```python
from build123d import *

# Parameters (mm, degrees)
SKETCH1_R           = 64
BOSS_EXTRUDE1_DEPTH = 7
SKETCH2_R           = 37.5
SKETCH2_R_2         = 32.5
BOSS_EXTRUDE2_DEPTH = 12
SKETCH3_R           = 12.5
CUT_EXTRUDE1_DEPTH  = 92.301697684
FILLET1_R           = 2
SKETCH17_R          = 13.5
BOSS_EXTRUDE3_DEPTH = 30


with BuildPart() as part:
    # Sketch1 → Boss-Extrude1 (new body)
    with BuildSketch(Plane(origin=(0, 0, 0), x_dir=(1, 0, 0), z_dir=(0, 1, 0))):
        with Locations(Location((0, 0, 0), (0, 0, 270))):
            Circle(SKETCH1_R)
    extrude(amount=BOSS_EXTRUDE1_DEPTH)

    # Sketch2 → Boss-Extrude2 (add)
    with BuildSketch(Plane(origin=(0, 7, 0), x_dir=(1, 0, 0), z_dir=(0, 1, 0))):
        with Locations(Location((0, 0, 0), (0, 0, 270))):
            Circle(SKETCH2_R)
        with Locations(Location((0, 0, 0), (0, 0, 270))):
            Circle(SKETCH2_R_2, mode=Mode.SUBTRACT)
    extrude(amount=BOSS_EXTRUDE2_DEPTH)

    # Sketch3 → Cut-Extrude1 (cut, through all)
    with BuildSketch(Plane(origin=(0, 7, 0), x_dir=(1, 0, 0), z_dir=(0, 1, 0))):
        with Locations(Location((0, 0, 0), (0, 0, 270))):
            Circle(SKETCH3_R)
    extrude(amount=-CUT_EXTRUDE1_DEPTH, mode=Mode.SUBTRACT)

    # Fillet1
    fillet1_edges = [part.edges().sort_by_distance(p)[0] for p in [
        (0, 0, -64),
        (0, 7, -64),
        (0, 19, -37.5),
        (0, 19, -32.5),
    ]]
    fillet(fillet1_edges, radius=FILLET1_R)

    # Sketch17 → Boss-Extrude3 (add)
    with BuildSketch(Plane(origin=(0, 7, 0), x_dir=(1, 0, 0), z_dir=(0, 1, 0))):
        with Locations(Location((0, 35, 0), (0, 0, 359.939369671))):
            Circle(SKETCH17_R)
    extrude(amount=BOSS_EXTRUDE3_DEPTH)


solid = part.part
```
Geometry: final body of the model. Coordinates: model frame, mm. A direction names the side the tool comes from. Round coordinates to 2 decimals unless told otherwise and drop trailing zeros. Write each loop counter-clockwise with the first axis right and the second up, starting at its lowest first coordinate (ties: lowest second). Pieces come first, ordered by that corner, then holes.
Item 1: Material intervals for L1, parallel to X at y = 11.75, z = 0; L2, parallel to X at y = 4.5, z = 0; L3, parallel to Y at x = 1, z = -53.5, sorted ascending.
Item 2: Set-up query: faces 4 (the face through (-27, 7, 27)), 5 (the face through (3.755, 3.549, 11.923)). Return all of +Z, -Z, +X, -X, +Y, -Y with unobstructed straight access to the full face (end or side cutting, diameter ignored); none if empty.
Item 3: Section query A-A (z = 0). Return loops of the section in (x, y).
Item 4: Section query C-C (y = 15). Return loops of the section in (x, z).
Item 5: Pin query (flat end, axial travel): P1, Ø10, axis at y = 10.5, z = 5, coming from the -X side; P2, Ø3, axis at x = -31, z = -50, coming from the +Y side; P3, Ø8, axis at x = -4, y = 14.5, coming from the -Z side. Return the tip coordinate at first contact, or that it passes through.
Item 6: Section query D-D (y = 28.5). Return loops of the section in (x, z).
Item 7: Section query B-B (x = 0). Return loops of the section in (y, z).
Item 8: Mould query, pull axis Z, two halves, no side actions, for faces 1 (the face through (-13, 0, -1)), 2 (the face through (-1.249, 11.93, 32.476)), 3 (the face through (-62.48, 3.48, -13.87)). Classes: +Z half, -Z half, draft (parallel to the pull), parting line (faces both ways), or undercut.
Completed:
1. L1: x = -37.5 to -32.5, 32.5 to 37.5
1. L2: x = -64 to -12.5, 12.5 to 64
1. L3: y = 0 to 7
2. face 4: +Y
2. face 5: +Y, -Y
3. outline: (-64, 2) arc R2 ccw to (-62, 0) - (-12.5, 0) - (-12.5, 7) - (-32.5, 7) - (-32.5, 17) arc R2 ccw to (-34.5, 19) - (-35.5, 19) arc R2 ccw to (-37.5, 17) - (-37.5, 7) - (-62, 7) arc R2 ccw to (-64, 5) - close; (12.5, 0) - (62, 0) arc R2 ccw to (64, 2) - (64, 5) arc R2 ccw to (62, 7) - (37.5, 7) - (37.5, 17) arc R2 ccw to (35.5, 19) - (34.5, 19) arc R2 ccw to (32.5, 17) - (32.5, 7) - (12.5, 7) - close
4. outline: (-13.5, -34.99) arc R13.5 ccw to (13.5, -34.99) arc R37.5 ccw (long way) to start; hole (-12.53, -29.99) arc R13.5 cw to (12.53, -29.99) arc R32.5 ccw (long way) to start
5. P1: stops at x = -63.78
5. P2: stops at y = 7
5. P3: stops at z = -48.5
6. outline: circle Ø27 at (0, -35)
7. outline: (0, -62) arc R2 ccw to (2, -64) - (5, -64) arc R2 ccw to (7, -62) - (7, -48.5) - (37, -48.5) - (37, -21.5) - (7, -21.5) - (7, -12.5) - (0, -12.5) - close; (0, 12.5) - (7, 12.5) - (7, 32.5) - (17, 32.5) arc R2 ccw to (19, 34.5) - (19, 35.5) arc R2 ccw to (17, 37.5) - (7, 37.5) - (7, 62) arc R2 ccw to (5, 64) - (2, 64) arc R2 ccw to (0, 62) - close
8. face 1: draft
8. face 2: undercut
8. face 3: parting line
